from build123d import *

# Parameters (mm, degrees)
SKETCH1_W           = 127
SKETCH1_H           = 139.7
BOSS_EXTRUDE5_DEPTH = 3.175
SKETCH2_R           = 5.0165
SKETCH2_R_2         = 1.5875
SKETCH2_R_3         = 4.7625
BOSS_EXTRUDE6_DEPTH = 6.35
CUT_EXTRUDE2_START  = -3.81
CUT_EXTRUDE2_DEPTH  = 3.81


with BuildPart() as part:
    # Sketch1 → Boss-Extrude5 (new body)
    with BuildSketch(Plane(origin=(0, 0, 0), x_dir=(1, 0, 0), z_dir=(0, 1, 0))):
        with Locations((63.5, -69.85)):
            Rectangle(SKETCH1_W, SKETCH1_H)
    extrude(amount=BOSS_EXTRUDE5_DEPTH)

    # Sketch2 → Boss-Extrude6 (add)
    # profile 1 of 10: a face of its own
    with BuildSketch(Plane(origin=(0, 3.175, 0), x_dir=(1, 0, 0), z_dir=(0, 1, 0))):
        with Locations(Location((12.3825, -15.84325, 0), (0, 0, 270))):
            Circle(SKETCH2_R)
        with Locations(Location((12.3825, -15.84325, 0), (0, 0, 270))):
            Circle(SKETCH2_R_2, mode=Mode.SUBTRACT)
    # profile 2 of 10: a face of its own
    with BuildSketch(Plane(origin=(0, 3.175, 0), x_dir=(1, 0, 0), z_dir=(0, 1, 0))):
        with Locations(Location((53.6575, -15.84325, 0), (0, 0, 270))):
            Circle(SKETCH2_R)
        with Locations(Location((53.6575, -15.84325, 0), (0, 0, 270))):
            Circle(SKETCH2_R_2, mode=Mode.SUBTRACT)
    # profile 3 of 10: a face of its own
    with BuildSketch(Plane(origin=(0, 3.175, 0), x_dir=(1, 0, 0), z_dir=(0, 1, 0))):
        with Locations(Location((71.755, -26.67, 0), (0, 0, 270))):
            Circle(SKETCH2_R_3)
        with Locations(Location((71.755, -26.67, 0), (0, 0, 270))):
            Circle(SKETCH2_R_2, mode=Mode.SUBTRACT)
    # profile 4 of 10: a face of its own
    with BuildSketch(Plane(origin=(0, 3.175, 0), x_dir=(1, 0, 0), z_dir=(0, 1, 0))):
        with Locations(Location((114.935, -25.527, 0), (0, 0, 270))):
            Circle(SKETCH2_R_3)
        with Locations(Location((114.935, -25.527, 0), (0, 0, 270))):
            Circle(SKETCH2_R_2, mode=Mode.SUBTRACT)
    # profile 5 of 10: a face of its own
    with BuildSketch(Plane(origin=(0, 3.175, 0), x_dir=(1, 0, 0), z_dir=(0, 1, 0))):
        with Locations(Location((104.14, -81.915, 0), (0, 0, 270))):
            Circle(SKETCH2_R_3)
        with Locations(Location((104.14, -81.915, 0), (0, 0, 270))):
            Circle(SKETCH2_R_2, mode=Mode.SUBTRACT)
    # profile 6 of 10: a face of its own
    with BuildSketch(Plane(origin=(0, 3.175, 0), x_dir=(1, 0, 0), z_dir=(0, 1, 0))):
        with Locations(Location((76.835, -81.915, 0), (0, 0, 270))):
            Circle(SKETCH2_R_3)
        with Locations(Location((76.835, -81.915, 0), (0, 0, 270))):
            Circle(SKETCH2_R_2, mode=Mode.SUBTRACT)
    # profile 7 of 10: a face of its own
    with BuildSketch(Plane(origin=(0, 3.175, 0), x_dir=(1, 0, 0), z_dir=(0, 1, 0))):
        with Locations(Location((53.6575, -81.94675, 0), (0, 0, 270))):
            Circle(SKETCH2_R)
        with Locations(Location((53.6575, -81.94675, 0), (0, 0, 270))):
            Circle(SKETCH2_R_2, mode=Mode.SUBTRACT)
    # profile 8 of 10: a face of its own
    with BuildSketch(Plane(origin=(0, 3.175, 0), x_dir=(1, 0, 0), z_dir=(0, 1, 0))):
        with Locations(Location((12.3825, -81.94675, 0), (0, 0, 270))):
            Circle(SKETCH2_R)
        with Locations(Location((12.3825, -81.94675, 0), (0, 0, 270))):
            Circle(SKETCH2_R_2, mode=Mode.SUBTRACT)
    # profile 9 of 10: a face of its own
    with BuildSketch(Plane(origin=(0, 3.175, 0), x_dir=(1, 0, 0), z_dir=(0, 1, 0))):
        with BuildLine():
            Line((15.24, -106.1339), (15.24, -101.8159))
            Line((15.24, -101.8159), (19.558, -101.8159))
            ThreePointArc((19.558, -101.8159), (21.717, -103.9749), (19.558, -106.1339))
            Line((19.558, -106.1339), (15.24, -106.1339))
        make_face()
    # profile 10 of 10: a face of its own
    with BuildSketch(Plane(origin=(0, 3.175, 0), x_dir=(1, 0, 0), z_dir=(0, 1, 0))):
        with BuildLine():
            Line((107.442, -101.8159), (111.76, -101.8159))
            Line((111.76, -101.8159), (111.76, -106.1339))
            Line((111.76, -106.1339), (107.442, -106.1339))
            ThreePointArc((107.442, -106.1339), (105.283, -103.9749), (107.442, -101.8159))
        make_face()
    extrude(amount=BOSS_EXTRUDE6_DEPTH)

    # Sketch3 → Cut-Extrude2 (cut)
    with BuildSketch(Plane(origin=(0, 9.525, 0), x_dir=(1, 0, 0), z_dir=(0, 1, 0)).offset(CUT_EXTRUDE2_START)):
        with BuildLine():
            Line((19.558, -101.8159), (15.24, -101.8159))
            Line((15.24, -101.8159), (15.24, -106.1339))
            Line((15.24, -106.1339), (19.558, -106.1339))
            ThreePointArc((19.558, -106.1339), (21.717, -103.9749), (19.558, -101.8159))
        make_face()
        with BuildLine():
            Line((111.76, -106.1339), (107.442, -106.1339))
            ThreePointArc((107.442, -106.1339), (105.283, -103.9749), (107.442, -101.8159))
            Line((107.442, -101.8159), (111.76, -101.8159))
            Line((111.76, -101.8159), (111.76, -106.1339))
        make_face()
    extrude(amount=CUT_EXTRUDE2_DEPTH, mode=Mode.SUBTRACT)


solid = part.part
For this review, take the finished solid that the model builds, in its own axes (mm). A direction names the side the tool comes from. Round coordinates to 2 decimals unless told otherwise and drop trailing zeros. Write each loop counter-clockwise with the first axis right and the second up, starting at its lowest first coordinate (ties: lowest second). Pieces come first, ordered by that corner, then holes. Notation, with made-up numbers: (28, 54) - (75, 54) arc R11 ccw to (75, 72) - close; hole circle Ø8 at (40.5, 27.25). An arc over 180 degrees is marked (long way). Use a Markdown table: item, result.
Q1. The part is to be moulded in two halves that separate along X. For faces 1 (the flat face through (18, 5.715, 104)), 2 (the flat face through (72, 3.175, 27)), say which applies: pulls with the +X half, pulls with the -X half, needs draft (parallel to the pull), parting line crosses it, or undercut.
Derived:
| item | result |
|---|---|
| face 1 | needs draft |
| face 2 | undercut |
Q2. We need section A-A (z = 65). Give the boundary of the cut face in (x, y) (3 decimals), plus the area to 3 significant figures.
Derived:
| item | result |
|---|---|
| outline | (0, 0) - (127, 0) - (127, 3.175) - (0, 3.175) - close |
| area | 403 mm2 |
Q3. Machinability: for faces 3 (the flat face through (63, 3.175, 69)), 4 (the flat face through (77, 9.525, 84)), which of the approach directions +Z, -Z, +X, -X, +Y, -Y give a long, thin tool a straight path to every point of the face, cutting with its end or side? Answer none if there is none.
Derived:
| item | result |
|---|---|
| face 3 | +Y |
| face 4 | +Z, -Z, +X, -X, +Y |
Q4. Clearance check with flat-ended pins moving along their axes: pin 1 (1.6 mm diameter, centred on x = 53.5, z = 15.5, fed in from +Y) (3 decimals); pin 2 (5 mm diameter, centred on y = 7.5, z = 22, fed in from +X); pin 3 (6 mm diameter, centred on x = 101, z = 40.5, fed in from -Y); pin 4 (2 mm diameter, centred on x = 18, z = 103, fed in from +Y) (3 decimals). State where each tip first meets the part, or that it passes through.
Derived:
| item | result |
|---|---|
| pin 1 | stops at y = 3.175 |
| pin 2 | stops at x = 119.59 |
| pin 3 | stops at y = 0 |
| pin 4 | stops at y = 5.715 |
Q5. We need section B-B (x = 62). Give the boundary of the cut face in (y, z) (3 decimals), plus the area to 3 significant figures.
Derived:
| item | result |
|---|---|
| outline | (0, 0) - (3.175, 0) - (3.175, 139.7) - (0, 139.7) - close |
| area | 444 mm2 |
Q6. Wall thickness on line 1 along X through (y, z) = (6, 28); line 2 along Y through (x, z) = (84, 100) (3 decimals); line 3 along Z through (x, y) = (105.5, 6.25): over which ranges is each line inside the solid? List them lowest first.
Derived:
| item | result |
|---|---|
| line 1 | x = 67.18 to 70.89, 72.62 to 76.33, 110.86 to 119.01 |
| line 2 | y = 0 to 3.175 |
| line 3 | z = 77.35 to 81.1, 82.73 to 86.48 |
